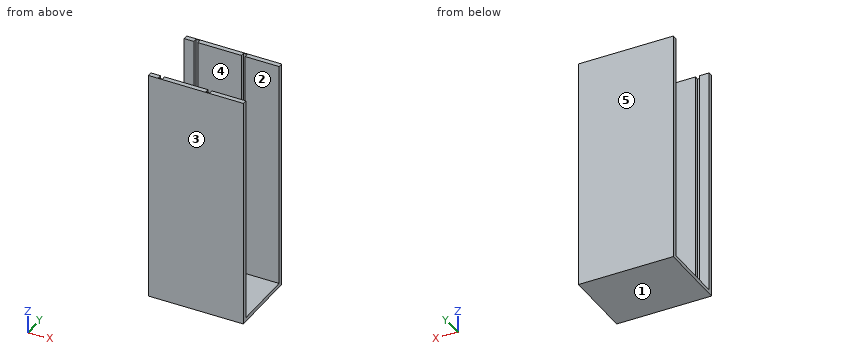
```python
from build123d import *

# Parameters (mm, degrees)
BOSS_EXTRUDE1_DEPTH   = 1500
BOSS_EXTRUDE1_2_DEPTH = 1500
SKETCH5_W             = 610
SKETCH5_H             = 460
BOSS_EXTRUDE5_DEPTH   = 25


with BuildPart() as part:
    # Sketch1 → Boss-Extrude1 (new body)
    with BuildSketch(Plane.XY):
        Polygon((0, -30), (217.5, -30), (217.5, -5), (242.5, -5), (242.5, -30), (460, -30), (460, 0), (0, 0), (-150, 0), (-150, -30), (-87.5, -30), (-87.5, -5), (-62.5, -5), (-62.5, -30), align=None)
    extrude(amount=BOSS_EXTRUDE1_DEPTH)



with BuildPart() as body_2:
    # Sketch1 → Boss-Extrude1 2 (new body)
    with BuildSketch(Plane.XY):
        Polygon((-62.5, -430), (0, -430), (217.5, -430), (217.5, -455), (242.5, -455), (242.5, -430), (460, -430), (460, -460), (0, -460), (-150, -460), (-150, -430), (-87.5, -430), (-87.5, -455), (-62.5, -455), align=None)
    extrude(amount=BOSS_EXTRUDE1_2_DEPTH)


with BuildPart() as part_1:
    add(part.part)

    add(body_2.part)  # Boss-Extrude5 merges body 2
    # Sketch5 → Boss-Extrude5 (add)
    with BuildSketch(Plane(origin=(0, 0, 0), x_dir=(-1, 0, 0), z_dir=(0, 0, -1))):
        with Locations((-155, -230)):
            Rectangle(SKETCH5_W, SKETCH5_H)
    extrude(amount=-BOSS_EXTRUDE5_DEPTH)


solid = part_1.part
```
Geometry check sheet. Reference: the model listing, model coordinates, mm. Face numbers are marked on the shaded views. A direction names the side the tool comes from. Give positions to 0.01 mm unless a question says otherwise; leave off trailing zeros. Loops run counter-clockwise (first coordinate to the right, second up) from the corner with the lowest first, then second, coordinate; pieces in that order, holes last. Notation, with made-up numbers: (59.5, 14) - (82.5, 14) arc R24 cw to (82.5, 42) - close; hole circle Ø10 at (-35.5, 40). An arc over 180 degrees is marked (long way). Use CSV: the item, a comma, the result in double quotes. Start each with the question number.
Q1. Section check C-C, the plane y = -49. Record the cut outline in (x, z), and give its area (4 significant figures).
Q2. Go/stop test with a flat-tipped pin: pin 1 Ø8 at (x, y) = (21, -219.5) entering from +Z. Record where the tip stops, or that it passes through.
Q3. Scan lines: probe 1 along Y at (x, z) = (30.5, 133.5); probe 2 along X at (y, z) = (-437, 422); probe 3 along Y at (x, z) = (241, 1223). Record each from-to range of solid material in increasing order. Write a range as from..to.
Q4. Section check B-B, the plane x = 362.5. Record the cut outline in (y, z), and give its area (3 significant figures).
Q5. Access from +Z, -Z, +X, -X, +Y, -Y to the whole of each face (thin tool, end or side, straight path). Record for the marked faces 4 and 5.
Q6. Release check for a two-part mould opening along Y. For the marked faces 1, 2 and 3 record: +Y half, -Y half, draft (parallel to the pull), parting line (faces both ways), or undercut.
Q7. Section check A-A, the plane z = 1263.5. Record the cut outline in (x, y), and give its area (3 significant figures).
Findings below:
1,outline,"(-150, 0) - (460, 0) - (460, 25) - (-150, 25) - close"
1,area,"15,250 mm^2"
2,pin 1,"stops at z = 25"
3,probe 1,"y = -460..-430, -30..0"
3,probe 2,"x = -150..-87.5, -62.5..217.5, 242.5..460"
3,probe 3,"y = -460..-455, -5..0"
4,outline,"(-460, 0) - (0, 0) - (0, 1500) - (-30, 1500) - (-30, 25) - (-430, 25) - (-430, 1500) - (-460, 1500) - close"
4,area,"100,000 mm^2"
5,face 4,"+Z, +X, -X"
5,face 5,"+Z, -Z, +X, -X, +Y"
6,face 1,"draft"
6,face 2,"undercut"
6,face 3,"-Y half"
7,outline,"(-150, -460) - (460, -460) - (460, -430) - (242.5, -430) - (242.5, -455) - (217.5, -455) - (217.5, -430) - (-62.5, -430) - (-62.5, -455) - (-87.5, -455) - (-87.5, -430) - (-150, -430) - close; (-150, -30) - (-87.5, -30) - (-87.5, -5) - (-62.5, -5) - (-62.5, -30) - (217.5, -30) - (217.5, -5) - (242.5, -5) - (242.5, -30) - (460, -30) - (460, 0) - (-150, 0) - close"
7,area,"34,100 mm^2"
